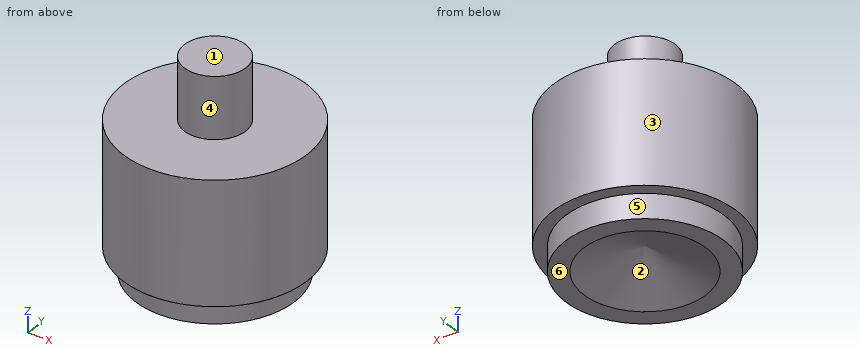
Autodesk Inventor part; units mm, degrees
ref_plane "YZ Plane" through (0, 0, 0) normal (1, 0, 0) x (0, 1, 0)
ref_plane "XZ Plane" through (0, 0, 0) normal (0, 1, 0) x (-1, 0, 0)
ref_plane "XY Plane" through (0, 0, 0) normal (0, 0, 1) x (1, 0, 0)
sketch "Sketch1" plane through (0, 0, 0) normal (0, 0, 1) x (1, 0, 0)
  circle A0 centre (0, 0) radius 7.5
  dimension "d0" = 15
extrude "Extrusion1" add sketch "Sketch1" along normal blind 10
sketch "Sketch2" plane through (0, 0, 0) normal (0, 0, -1) x (-1, 0, 0)
  circle A0 centre (0, 0) radius 6.5
  circle A1 centre (0, 0) radius 5
  circle A2 centre (0, 0) radius 7.5
  dimension "d3" = 13
  dimension "d4" = 15
  dimension "d5" = 10
extrude "Extrusion2" add sketch "Sketch2" along normal blind 2 contours A0
sketch "Sketch3" plane through (0, 0, 10) normal (0, 0, 1) x (1, 0, 0)
  circle A0 centre (0, 0) radius 7.5
  circle A1 centre (0, 0) radius 2.5
  dimension "d8" = 15
  dimension "d13" = 5
extrude "Extrusion3" add sketch "Sketch3" along normal blind 5 contours A1
chamfer "Chamfer1" distance 2 angle 68.199 1 edges at (5, 0, 0) measured on face at (-4.9838, -0.4023, -1.3333)
properties part number "stredne_koleso"
Verification items for the finished model (mm, model axes). Face numbers are marked on the shaded views. A direction names the side the tool comes from. Coordinates: 2 decimals unless noted, no trailing zeros. Write each loop counter-clockwise with the first axis right and the second up, starting at its lowest first coordinate (ties: lowest second). Pieces come first, ordered by that corner, then holes. Notation, with made-up numbers: M 19,49.25 L 46,49.25 A25 cw 46,85.25 Z; hole C 55.5,-33 d6. An arc over 180 degrees is marked long. Use a Markdown table: item, result.
Q1. Set-up check for the marked faces 4, 5 and 6: record each of +Z, -Z, +X, -X, +Y, -Y from which the full face is reachable in a straight line by a thin tool's end or side.
Reply:
| item | result |
|---|---|
| face 4 | +Z |
| face 5 | -Z |
| face 6 | -Z, +X, -X, +Y, -Y |
Q2. Draft check along X on the marked faces 1, 2 and 3. Enter one of: +X half, -X half, draft (parallel to the pull), parting line (faces both ways), or undercut.
Reply:
| item | result |
|---|---|
| face 1 | draft |
| face 2 | undercut |
| face 3 | parting line |
Q3. Go/stop test with flat-tipped pins: P1, Ø1, axis at y = 3, z = 2, coming from the -X side; P2, Ø9, axis at x = 0, y = 0, coming from the -Z side; P3, Ø6, axis at x = -3, y = 0, coming from the -Z side; P4, Ø4, axis at x = 4, z = 11.5, coming from the +Y side. Record where each tip stops, or that it passes through.
Reply:
| item | result |
|---|---|
| P1 | stops at x = -7.07 |
| P2 | stops at z = -1.8 |
| P3 | stops at z = -2 |
| P4 | stops at y = 7.01 |
Q4. Sectioned sample at C-C, the plane z = 10.5. Record the boundary of the cut face in (x, y), plus the area to 3 significant figures.
Reply:
| item | result |
|---|---|
| outline | C 0,0 d5 |
| area | 19.6 mm² |
Q5. Sectioned sample at B-B, the plane z = 0.25. Record the boundary of the cut face in (x, y), plus the area to 3 significant figures.
Reply:
| item | result |
|---|---|
| outline | C 0,0 d15 |
| area | 177 mm² |
Q6. Thickness scan on line 1 (Z direction, x = 6, y = 2); line 2 (Z direction, x = -7, y = -2.25); line 3 (Y direction, x = 4.75, z = 2.25). Record the ranges inside material, lowest first.
Reply:
| item | result |
|---|---|
| line 1 | z = -2 to 10 |
| line 2 | z = 0 to 10 |
| line 3 | y = -5.8 to 5.8 |
Q7. Sectioned sample at A-A, the plane x = -5.5. Record the boundary of the cut face in (y, z).
Reply:
| item | result |
|---|---|
| outline | M -5.1,0 L -3.46,0 L -3.46,-2 L 3.46,-2 L 3.46,0 L 5.1,0 L 5.1,10 L -5.1,10 Z |
